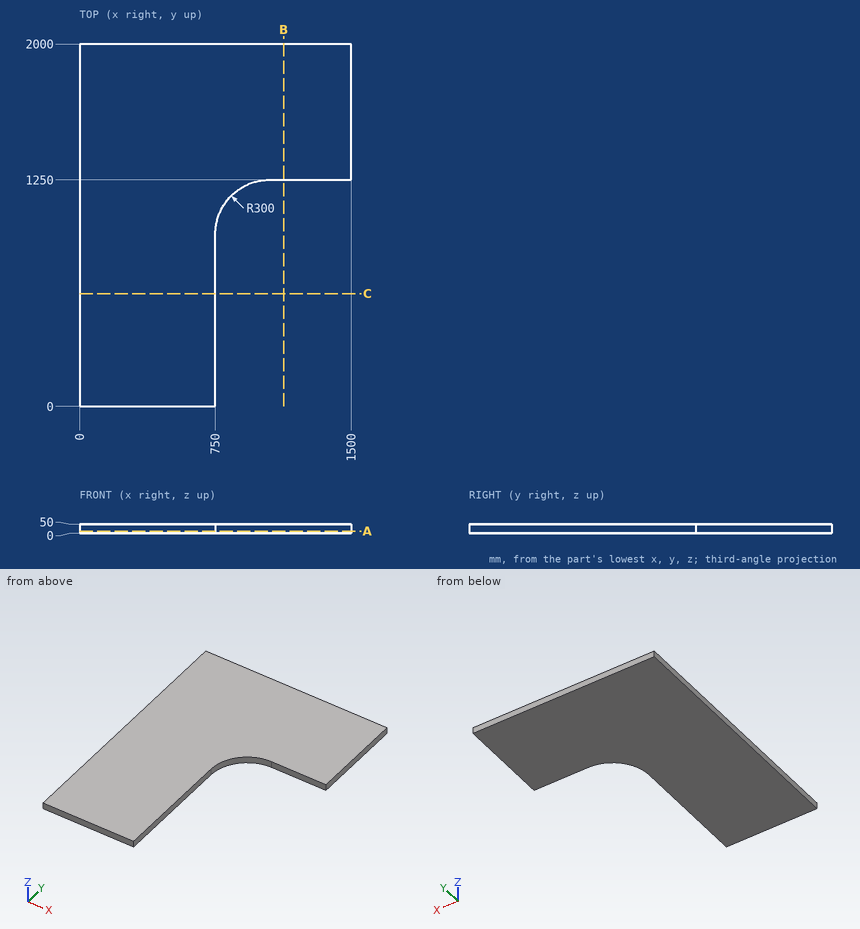
Here's the drawing with two shaded views (mm, measured from the low corner). I have some questions. Give positions to 0.01 mm unless a question says otherwise; leave off trailing zeros. Loops run counter-clockwise (first coordinate to the right, second up) from the corner with the lowest first, then second, coordinate; pieces in that order, holes last. Notation, with made-up numbers: (-17, -33) -> (12, -33) arc R17 cw to (12, -6) -> close; hole circle Ø6 at (67.5, 22). An arc over 180 degrees is marked (long way). Use one line per item in the form item = value.
1) If we section it at A-A (z = 12): Please give me the cut outline in (x, y), plus the area to 3 significant figures.
Answers:
outline = (0, 0) -> (750, 0) -> (750, 950) arc R300 cw to (1050, 1250) -> (1500, 1250) -> (1500, 2000) -> (0, 2000) -> close
area = 2,080,000 mm²
2) If we section it at C-C (y = 621.5): Please give me the cut outline in (x, z).
Answers:
outline = (0, 0) -> (750, 0) -> (750, 50) -> (0, 50) -> close
3) Will these pins go through, and if not, where does the flat tip stop? pin 1 (8 mm diameter, centred on x = 1347.5, z = 38.5, fed in from -Y); pin 2 (10 mm diameter, centred on y = 1084.5, z = 44, fed in from +X); pin 3 (6 mm diameter, centred on y = 693, z = 11, fed in from +X).
Answers:
pin_1 = 1250
pin_2 = 784.41
pin_3 = 750
4) If we section it at B-B (x = 1126.5): Please give me the cut outline in (y, z), plus the area to 3 significant figures.
Answers:
outline = (1250, 0) -> (2000, 0) -> (2000, 50) -> (1250, 50) -> close
area = 37,500 mm²
5) I need wall thicknesses on line 1 along Y through (x, z) = (1427, 12); line 2 along X through (y, z) = (928.5, 16); line 3 along X through (y, z) = (958, 12). Which ranges of each line are inside material? Lowest first, please.
Answers:
line_1 = 1250 to 2000
line_2 = 0 to 750
line_3 = 0 to 750.11
